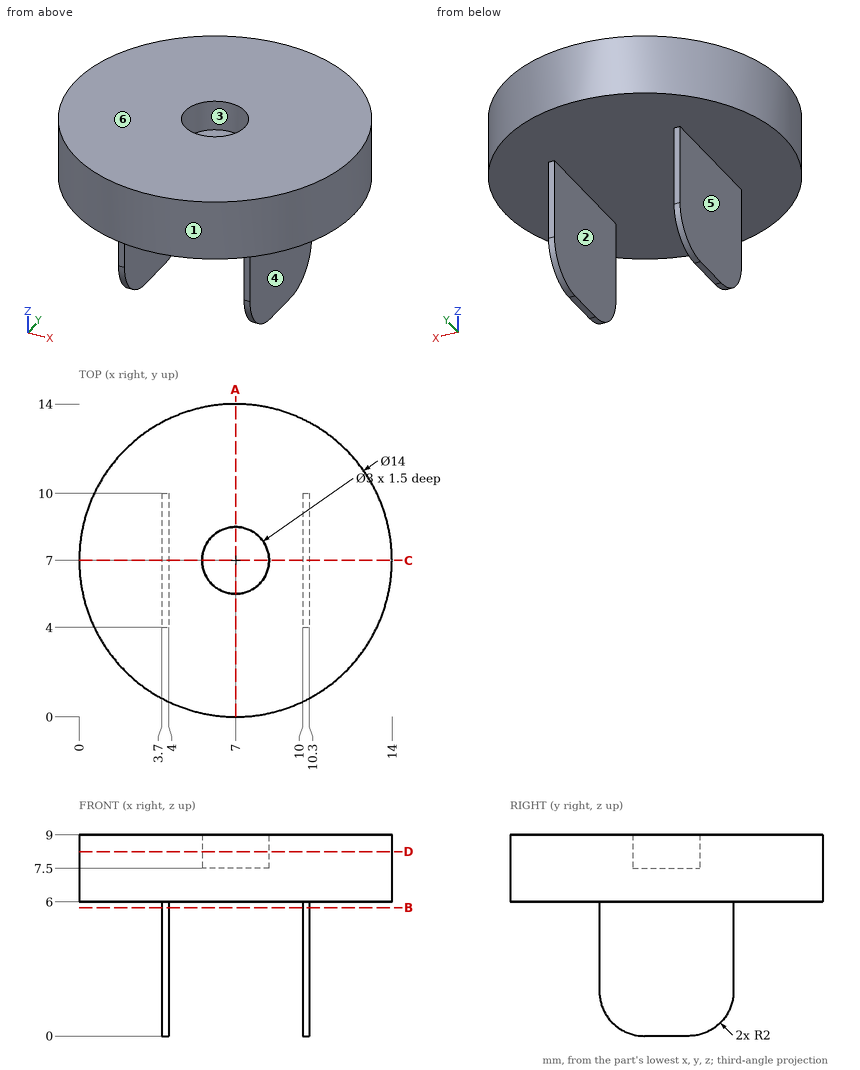
Verification items for this drawing (mm, ordinates from the low corner). A direction names the side the tool comes from. Coordinates: 2 decimals unless noted, no trailing zeros. Order: outer loops, then holes, each group sorted by start corner. A loop starts at its lowest first (then second) coordinate and runs counter-clockwise, first axis right, second up.
Q1. Tool access check on the marked faces 1 and 2. Record the directions out of +Z, -Z, +X, -X, +Y, -Y that give a thin tool (end or side, any length) a straight path to the whole face; none if there is none.
Reply:
face 1: +Z, -Z
face 2: -Z, +Y, -Y
Q2. Draft check along X on the marked faces 3, 4, 5 and 6. Enter one of: released by +X, released by -X, zero draft, split by the parting line, or undercut.
Reply:
face 3: undercut
face 4: released by +X
face 5: released by -X
face 6: zero draft
Q3. Sectioned sample at B-B on z = 5.75. Record the cut outline in (x, y).
Reply:
outline: (3.7, 4) - (4, 4) - (4, 10) - (3.7, 10) - close; (10, 4) - (10.3, 4) - (10.3, 10) - (10, 10) - close
Q4. Depth check by flat-ended pin: pin 1 Ø1.8 at (y, z) = (7.5, 2) entering from -X; pin 2 Ø1 at (y, z) = (4.5, 6) entering from -X; pin 3 Ø2 at (x, z) = (8.5, 7) entering from +Y. Enter the tip coordinate at first touch or a pass-through.
Reply:
pin 1: stops at x = 3.7
pin 2: stops at x = 0.29
pin 3: stops at y = 13.98
Q5. Sectioned sample at A-A on x = 7. Record the cut outline in (y, z), and give its area (3 significant figures).
Reply:
outline: (0, 6) - (14, 6) - (14, 9) - (8.5, 9) - (8.5, 7.5) - (5.5, 7.5) - (5.5, 9) - (0, 9) - close
area: 37.5 mm2
Q6. Thickness scan on probe 1 along Y at (x, z) = (7, 8.5); probe 2 along Z at (x, y) = (2, 4); probe 3 along X at (y, z) = (9.5, 2.75). Record the ranges inside material, lowest first.
Reply:
probe 1: y = 0 to 5.5, 8.5 to 14
probe 2: z = 6 to 9
probe 3: x = 3.7 to 4, 10 to 10.3
Q7. Sectioned sample at D-D on z = 8.25. Record the cut outline in (x, y).
Reply:
outline: circle Ø14 at (7, 7); hole circle Ø3 at (7, 7)
Q8. Sectioned sample at C-C on y = 7. Record the cut outline in (x, z), and give its area (3 significant figures).
Reply:
outline: (0, 6) - (3.7, 6) - (3.7, 0) - (4, 0) - (4, 6) - (10, 6) - (10, 0) - (10.3, 0) - (10.3, 6) - (14, 6) - (14, 9) - (8.5, 9) - (8.5, 7.5) - (5.5, 7.5) - (5.5, 9) - (0, 9) - close
area: 41.1 mm2
